Autodesk Inventor part; units mm, degrees
ref_plane "YZ Plane" through (0, 0, 0) normal (1, 0, 0) x (0, 1, 0)
ref_plane "XZ Plane" through (0, 0, 0) normal (0, 1, 0) x (-1, 0, 0)
ref_plane "XY Plane" through (0, 0, 0) normal (0, 0, 1) x (1, 0, 0)
sketch "Sketch1" plane through (0, 0, 0) normal (0, 0, 1) x (1, 0, 0)
  line L0 (0, 0) -> (27, 0)
  line L1 (27, 0) -> (27, 13.5)
  line L2 (27, 13.5) -> (0, 13.5)
  line L3 (0, 13.5) -> (0, 0)
  line L4 (13.4862, 18.9079) -> (13.4862, -5.216) construction
  line L5 (13.4862, -5.216) -> (23.4862, -5.216) construction
  line L6 (23.4862, -5.216) -> (23.4862, 20) construction
  line L7 (23.4862, 20) -> (3.4862, 20) construction
  line L8 (3.4862, 20) -> (3.4862, -7.3205) construction
  line L9 (14, 12) -> (14, 9) construction
  line L10 (13.5, 13.5) -> (13.5, 8.6504) construction
  line L11 (13.5, 8.6504) -> (13.5, 6.3397) construction
  line L12 (-7, 6.846) -> (36, 6.846) construction
  point P0 (3.4862, 6.846)
  point P1 (23.4862, 6.846)
  dimension "d0" = 27
  dimension "d1" = 13.5
  dimension "d2" = 10
  dimension "d3" = 20
extrude "Extrusion1" add sketch "Sketch1" along normal blind 2
hole "Hole1" at (3.4862, 6.846, 0) at (23.4862, 6.846, 0) direction (0, 0, 1) diameter 3.5 end through all
sketch "Sketch2" plane through (0, 0, 2) normal (0, 0, 1) x (1, 0, 0)
  circle A0 centre (3.4862, 6.846) radius 1.75
  circle A1 centre (23.4862, 6.846) radius 1.75
  line L0 (5, 5) -> (2.6444, 4.6119)
  line L1 (2.6444, 4.6119) -> (1.1306, 6.4579)
  line L2 (1.1306, 6.4579) -> (1.9723, 8.6919)
  line L3 (1.9723, 8.6919) -> (4.3279, 9.08)
  line L4 (4.3279, 9.08) -> (5.8417, 7.234)
  line L5 (5.8417, 7.234) -> (5, 5)
  line L6 (24.3353, 4.6119) -> (21.976, 4.9936)
  line L7 (21.976, 4.9936) -> (21.1269, 7.2276)
  line L8 (21.1269, 7.2276) -> (22.637, 9.08)
  line L9 (22.637, 9.08) -> (24.9963, 8.6983)
  line L10 (24.9963, 8.6983) -> (25.8454, 6.4643)
  line L11 (25.8454, 6.4643) -> (24.3353, 4.6119)
extrude "Extrusion2" cut sketch "Sketch2" against normal blind 1 contours L0 L1 L2 L3 L4 L5
extrude "Extrusion3" cut sketch "Sketch2" against normal blind 1 contours L6 L7 L8 L9 L10 L11
sketch "Sketch4" plane through (0, 0, 0) normal (0, 1, 0) x (-1, 0, 0)
  line L0 (-6.7373, -10.6634) -> (-6.7373, -4.6634) construction
  line L1 (-27, -7.5) -> (0, -7.5) construction
  line L2 (0, -7.5) -> (-27, -7.5) construction
  line L3 (-13.5, -7.5) -> (-13.5, 2) construction
  arc A0 (-9.2574, 2) -> (-17.7426, 2) centre (-13.5, 10.5) ccw
  circle A1 centre (-13.5, 10.5) radius 8.25
  line L4 (-9.2574, 2) -> (-17.7426, 2)
  point P0 (0, 0)
  dimension "d17" = 9.5
  dimension "d18" = 19
  dimension "d19" = 16.5
extrude "Extrusion4" add sketch "Sketch4" along normal blind 13.5
sketch "Sketch5" plane through (0, 0, 0) normal (0, -1, 0) x (1, 0, 0)
  circle A0 centre (13.5, 10.5) radius 8.25
  circle A1 centre (13.5, 10.5) radius 6
  circle A2 centre (13.5, 10.5) radius 8.25
  dimension "d22" = 12
extrude "Extrusion5" add sketch "Sketch5" against normal blind 1
properties part number "bart xl rjmp 2 part bearing holder v6"
CAD build for the part. Positions are in the model's coordinates, mm. A direction names the side the tool comes from. Give positions to 0.01 mm unless a question says otherwise; leave off trailing zeros. Loops run counter-clockwise (first coordinate to the right, second up) from the corner with the lowest first, then second, coordinate; pieces in that order, holes last. Notation, with made-up numbers: M 15,4.5 L 71,4.5 A34 cw 71,38.5 Z; hole C 89.5,-39 d10. An arc over 180 degrees is marked long. Use one line per item in the form item = value.
Item 1: Which spindle directions (+Z, -Z, +X, -X, +Y, -Y) get a long thin tool onto all of the face, cutting with end or side? Do faces 1 (the face through (21.56, 6.09, 1.51)), 2 (the face through (3.4, 5.1, 0.5)), 3 (the face through (1.546, 7.559, 1.507)). Say none if no direction does.
Determined:
face_1 = none
face_2 = -Z
face_3 = +Z
Item 2: Slice it at A-A (z = 10.5). List the corners of the cut face in (x, y), plus the area to 3 significant figures.
Determined:
outline = M 4,0 L 7.5,0 L 7.5,1 L 5.25,1 L 5.25,13.5 L 4,13.5 Z; M 19.5,0 L 23,0 L 23,13.5 L 21.75,13.5 L 21.75,1 L 19.5,1 Z
area = 38.2 mm2
Item 3: Flat gauge pins, fed straight in: pin 1 (2 mm diameter, centred on x = 14.5, z = 4, fed in from -Y); pin 2 (4 mm diameter, centred on x = 8.5, z = 14, fed in from +Y); pin 3 (6 mm diameter, centred on y = 12, z = 10, fed in from +X); pin 4 (5 mm diameter, centred on x = 3.5, y = 7.5, fed in from +Z). Where does each tip first touch, or does it go through?
Determined:
pin_1 = 0
pin_2 = 1
pin_3 = 23
pin_4 = 16.33
Item 4: Slice it at D-D (z = 17). List the corners of the cut face in (x, y).
Determined:
outline = M 6.57,0 L 20.43,0 L 20.43,13.5 L 18.58,13.5 L 18.58,1 L 8.42,1 L 8.42,13.5 L 6.57,13.5 Z
Item 5: Two-plate mould, pull along Y, no slides. Class faces 4 (the face through (19.04, 0.49, 8.2)), 5 (the face through (14, 1, 4)), 6 (the face through (5.427, 6.133, 1.507)): pulls with the +Y half, pulls with the -Y half, needs draft (parallel to the pull), parting line crosses it, or undercut.
Determined:
face_4 = needs draft
face_5 = pulls with the +Y half
face_6 = undercut
Item 6: Slice it at C-C (x = 13.5). List the corners of the cut face in (y, z).
Determined:
outline = M 0,0 L 13.5,0 L 13.5,2.25 L 1,2.25 L 1,4.5 L 0,4.5 Z; M 0,16.5 L 1,16.5 L 1,18.75 L 13.5,18.75 L 13.5,20 L 0,20 Z
Item 7: Slice it at B-B (y = 4.25). List the corners of the cut face in (x, z).
Determined:
outline = M 0,0 L 27,0 L 27,2 L 17.74,2 A9.5 ccw long 9.26,2 L 0,2 Z; hole C 13.5,10.5 d16.5
Item 8: Drill centre lines: probe 1 along Z at (x, y) = (13.5, 0.7); probe 2 along Z at (x, y) = (13.5, 8); probe 3 along Z at (x, y) = (1.75, 4.5). Where is each one in solid material? Low to high. Write a range as from..to.
Determined:
probe_1 = 0..4.5, 16.5..20
probe_2 = 0..2.25, 18.75..20
probe_3 = 0..2
